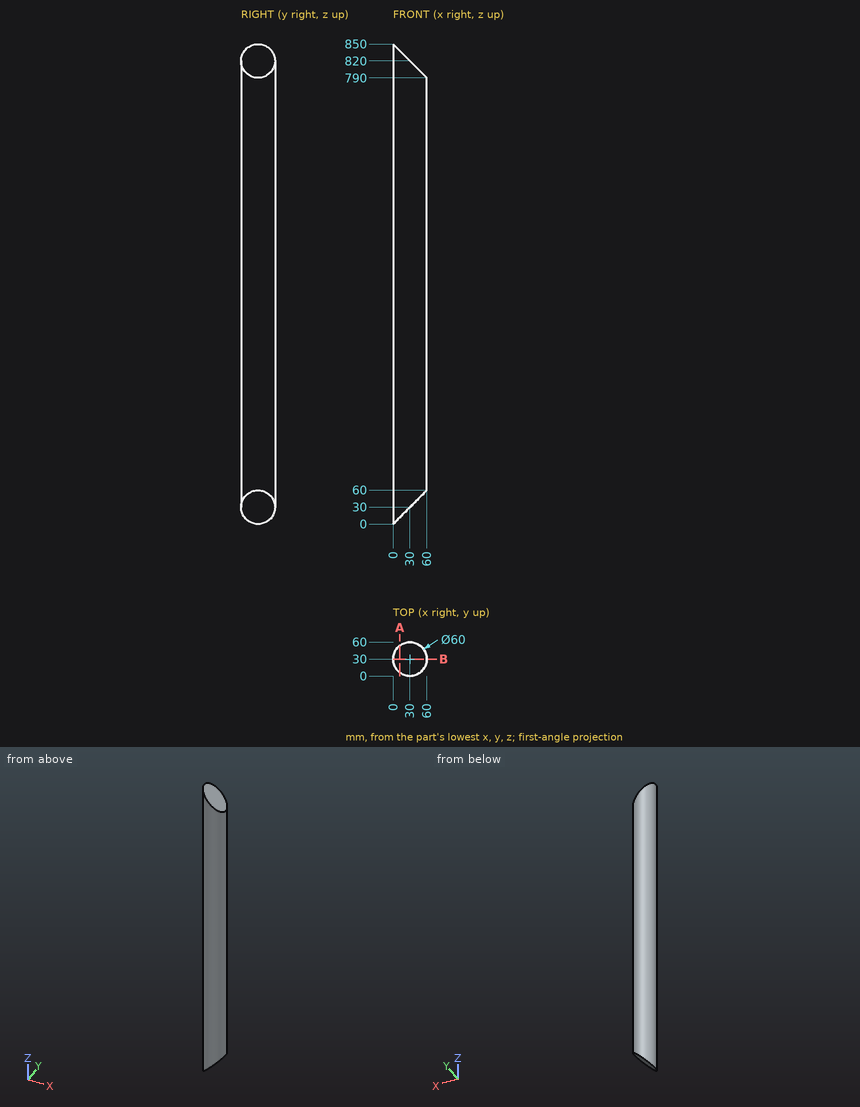
Input: dimensioned drawing with shaded views. Units: mm. Origin: part minimum x, y, z. Give positions to 0.01 mm unless a question says otherwise; leave off trailing zeros. Write each loop counter-clockwise with the first axis right and the second up, starting at its lowest first coordinate (ties: lowest second). Pieces come first, ordered by that corner, then holes. Notation, with made-up numbers: (11.25, -29) -> (56.25, -29) arc R16 ccw to (56.25, -23) -> close; hole circle Ø4 at (0, 24). An arc over 180 degrees is marked (long way). Return JSON: item names as keys, results as strings. Group by question number.
1. Section B-B, the plane y = 30. Output: boundary loops of the cut face in (x, z).
2. Material intervals for line 1 (X direction, y = 31, z = 257); line 2 (X direction, y = 10.5, z = 510); line 3 (Y direction, x = 20.5, z = 799.5), sorted ascending. Write a range as from..to.
3. Section A-A, the plane x = 12. Output: boundary loops of the cut face in (y, z).
4. Pin query (flat end, axial travel): pin 1 Ø12 at (y, z) = (11.5, 360) entering from -X; pin 2 Ø3 at (x, y) = (18.5, 24.5) entering from -Z; pin 3 Ø2 at (x, z) = (26.5, 163.5) entering from +Y. Return the tip coordinate at first contact, or that it passes through.
Determined:
{
 "1": {"outline": "(0, 0) -> (60, 60) -> (60, 790) -> (0, 850) -> close"},
 "2": {"line 1": "x = 0.02..59.98", "line 2": "x = 7.2..52.8", "line 3": "y = 1.54..58.46"},
 "3": {"outline": "(6, 12) -> (54, 12) -> (54, 838) -> (6, 838) -> close"},
 "4": {"pin 1": "stops at x = 2.73", "pin 2": "stops at z = 17", "pin 3": "stops at y = 59.9"}
}
